```python
from build123d import *

# Parameters (mm, degrees)
SKETCH_1_R          = 7
SKETCH_1_R_2        = 4
EXTRUDE_1_DEPTH     = 4
SKETCH_2_R          = 6.5
SKETCH_2_R_2        = 4.5
CUT_EXTRUDE_1_DEPTH = 0.2
SKETCH_3_R          = 6.5
SKETCH_3_R_2        = 4.5
CUT_EXTRUDE_2_DEPTH = 0.2


with BuildPart() as part:
    # 草图1 → 凸台-拉伸1 (new body)
    with BuildSketch(Plane(origin=(0, 0, 0), x_dir=(0, 0, -1), z_dir=(1, 0, 0))):
        Circle(SKETCH_1_R)
        Circle(SKETCH_1_R_2, mode=Mode.SUBTRACT)
    extrude(amount=EXTRUDE_1_DEPTH)

    # 草图2 → 切除-拉伸1 (cut)
    with BuildSketch(Plane(origin=(4, 0, 0), x_dir=(0, 0, -1), z_dir=(1, 0, 0))):
        Circle(SKETCH_2_R)
        Circle(SKETCH_2_R_2, mode=Mode.SUBTRACT)
    extrude(amount=-CUT_EXTRUDE_1_DEPTH, mode=Mode.SUBTRACT)

    # 草图3 → 切除-拉伸2 (cut)
    with BuildSketch(Plane.ZY):
        Circle(SKETCH_3_R)
        Circle(SKETCH_3_R_2, mode=Mode.SUBTRACT)
    extrude(amount=-CUT_EXTRUDE_2_DEPTH, mode=Mode.SUBTRACT)


solid = part.part
```
Verification items for the finished model (mm, model axes). A direction names the side the tool comes from. Give positions to 0.01 mm unless a question says otherwise; leave off trailing zeros. Order: outer loops, then holes, each group sorted by start corner. A loop starts at its lowest first (then second) coordinate and runs counter-clockwise, first axis right, second up. Notation, with made-up numbers: (-31.75, -21) -> (-21.75, -21) arc R24 cw to (-21.75, -8) -> close; hole circle Ø5 at (6.5, 22.5). An arc over 180 degrees is marked (long way). Use a Markdown table: item, result.
1) Depth check by flat-ended pin: pin 1 Ø3 at (y, z) = (-4, -5) entering from -X; pin 2 Ø1.5 at (x, z) = (1.5, 4.5) entering from -Y. Enter the tip coordinate at first touch or a pass-through.
Results:
| item | result |
|---|---|
| pin 1 | x = 0 |
| pin 2 | y = -5.91 |
2) Tool access check on faces 4 (the flat face through (0.2, 1.54, -4.42)), 5 (the cylindrical face through (1.972, -3.905, 0.867)). Record the directions out of +Z, -Z, +X, -X, +Y, -Y that give a thin tool (end or side, any length) a straight path to the whole face; none if there is none.
Results:
| item | result |
|---|---|
| face 4 | -X |
| face 5 | +X, -X |
3) Section check C-C, the plane x = 0.5. Record the boundary of the cut face in (y, z), then the cut area to 3 significant figures.
Results:
| item | result |
|---|---|
| outline | circle Ø14 at (0, 0); hole circle Ø8 at (0, 0) |
| area | 104 mm² |
4) Section check A-A, the plane y = 0. Record the boundary of the cut face in (x, z).
Results:
| item | result |
|---|---|
| outline | (0, -7) -> (4, -7) -> (4, -6.5) -> (3.8, -6.5) -> (3.8, -4.5) -> (4, -4.5) -> (4, -4) -> (0, -4) -> (0, -4.5) -> (0.2, -4.5) -> (0.2, -6.5) -> (0, -6.5) -> close; (0, 4) -> (4, 4) -> (4, 4.5) -> (3.8, 4.5) -> (3.8, 6.5) -> (4, 6.5) -> (4, 7) -> (0, 7) -> (0, 6.5) -> (0.2, 6.5) -> (0.2, 4.5) -> (0, 4.5) -> close |
5) Material ranges on probe 1 along Y at (x, z) = (0.1, 0); probe 2 along Y at (x, z) = (2.45, 0); probe 3 along X at (y, z) = (0.5, -6.25), recorded low to high.
Results:
| item | result |
|---|---|
| probe 1 | -7 to -6.5, -4.5 to -4, 4 to 4.5, 6.5 to 7 |
| probe 2 | -7 to -4, 4 to 7 |
| probe 3 | 0.2 to 3.8 |
6) Section check D-D, the plane z = 5.5. Record the boundary of the cut face in (x, y).
Results:
| item | result |
|---|---|
| outline | (0, -4.33) -> (4, -4.33) -> (4, -3.46) -> (3.8, -3.46) -> (3.8, 3.46) -> (4, 3.46) -> (4, 4.33) -> (0, 4.33) -> (0, 3.46) -> (0.2, 3.46) -> (0.2, -3.46) -> (0, -3.46) -> close |
7) Mould release check, pull along Z, two halves, no side actions. Record for faces 1 (the flat face through (3.8, 1.54, 4.42)), 2 (the cylindrical face through (1.972, -2.681, -6.466)), 3 (the flat face through (0, -3, 3)): pulls with the +Z half, pulls with the -Z half, needs draft (parallel to the pull), parting line crosses it, or undercut.
Results:
| item | result |
|---|---|
| face 1 | undercut |
| face 2 | parting line crosses it |
| face 3 | needs draft |
